Check sheet for the modelled part. Datum: model origin and axes. Units: mm. A direction names the side the tool comes from. Give positions to 0.01 mm unless a question says otherwise; leave off trailing zeros. Order: outer loops, then holes, each group sorted by start corner. A loop starts at its lowest first (then second) coordinate and runs counter-clockwise, first axis right, second up.
```python
from build123d import *

# Parameters (mm, degrees)
BOSS_EXTRUDE1_DEPTH     = 870
SKETCH3_W               = 20
SKETCH3_H               = 20
CUT_EXTRUDE1_DEPTH      = 1040.5
CUT_EXTRUDE6_DEPTH      = 871.675140337
CUT_EXTRUDE6_DEPTH_BACK = 871.675140337


with BuildPart() as part:
    # Sketch1 → Boss-Extrude1 (new body)
    with BuildSketch(Plane(origin=(0, 0, 0), x_dir=(1, 0, 0), z_dir=(0, 1, 0))):
        with BuildLine():
            Line((2.8, 0), (22.8, 0))
            ThreePointArc((22.8, 0), (24.779898987, -0.820101013), (25.6, -2.8))
            Line((25.6, -2.8), (25.6, -22.8))
            ThreePointArc((25.6, -22.8), (24.779898987, -24.779898987), (22.8, -25.6))
            Line((22.8, -25.6), (2.8, -25.6))
            ThreePointArc((2.8, -25.6), (0.820101013, -24.779898987), (0, -22.8))
            Line((0, -22.8), (0, -2.8))
            ThreePointArc((0, -2.8), (0.820101013, -0.820101013), (2.8, 0))
        make_face()
    extrude(amount=BOSS_EXTRUDE1_DEPTH)

    # Sketch3 → Cut-Extrude1 (cut)
    with BuildSketch(Plane(origin=(0, 0, 0), x_dir=(-1, 0, 0), z_dir=(0, -1, 0))):
        with Locations((-12.8, -12.8)):
            Rectangle(SKETCH3_W, SKETCH3_H)
    extrude(amount=-CUT_EXTRUDE1_DEPTH, mode=Mode.SUBTRACT)

    # Sketch4 → Cut-Extrude6 (cut, two sides: drawn at the far end of the back side and taken through both)
    with BuildSketch(Plane(origin=(0, 0, 22.8), x_dir=(-1, 0, 0), z_dir=(0, 0, -1)).offset(-CUT_EXTRUDE6_DEPTH_BACK)):
        Polygon((1655.369600379, 1439.989463611), (0, 870), (-25.6, 861.1852131), (-1680.969600379, 291.195749489), (-2820.948527601, 3601.934950248), (515.390673158, 4750.728664369), align=None)
    extrude(amount=CUT_EXTRUDE6_DEPTH + CUT_EXTRUDE6_DEPTH_BACK, mode=Mode.SUBTRACT)


solid = part.part
```
(1) Cross-section at C-C on x = 16. Enter the section's corners in (y, z), then the cut area to 3 significant figures.
Response values:
outline: (0, 0) - (864.49, 0) - (864.49, 2.8) - (0, 2.8) - close; (0, 22.8) - (864.49, 22.8) - (864.49, 25.6) - (0, 25.6) - close
area: 4,840 mm2
(2) Release check for a two-part mould opening along X. For faces 1 (the face through (12.621, 865.654, 1.601)), 2 (the face through (2.8, 428, 13)), 3 (the face through (13, 428, 0)), 4 (the face through (0, 429, 13)) record: released by +X, released by -X, zero draft, split by the parting line, or undercut.
Response values:
face 1: released by +X
face 2: undercut
face 3: zero draft
face 4: released by -X
(3) Cross-section at B-B on y = 364. Enter the section's corners in (x, z).
Response values:
outline: (0, 2.8) arc R2.8 ccw to (2.8, 0) - (22.8, 0) arc R2.8 ccw to (25.6, 2.8) - (25.6, 22.8) arc R2.8 ccw to (22.8, 25.6) - (2.8, 25.6) arc R2.8 ccw to (0, 22.8) - close; hole (2.8, 2.8) - (22.8, 2.8) - (22.8, 22.8) - (2.8, 22.8) - close
(4) Set-up check for faces 5 (the face through (13, 428, 25.6)), 6 (the face through (13, 428, 2.8)): record each of +Z, -Z, +X, -X, +Y, -Y from which the full face is reachable in a straight line by a thin tool's end or side.
Response values:
face 5: +Z, +X, -X, +Y, -Y
face 6: +Y, -Y
(5) Material ranges on L1, parallel to X at y = 666, z = 22.75; L2, parallel to Z at x = 23.25, y = 731.5, recorded low to high.
Response values:
L1: x = 0 to 2.8, 22.8 to 25.6
L2: z = 0.04 to 25.56
(6) Cross-section at A-A on z = 18.25. Enter the section's corners in (x, y), then the cut area to 3 significant figures.
Response values:
outline: (0, 0) - (2.8, 0) - (2.8, 869.04) - (0, 870) - close; (22.8, 0) - (25.6, 0) - (25.6, 861.19) - (22.8, 862.15) - close
area: 4,850 mm2
